Can you work these out from the drawing? Everything is in mm from the part's minimum corner. A direction names the side the tool comes from. Give positions to 0.01 mm unless a question says otherwise; leave off trailing zeros. Write each loop counter-clockwise with the first axis right and the second up, starting at its lowest first coordinate (ties: lowest second). Pieces come first, ordered by that corner, then holes. Notation, with made-up numbers: (34, -33) -> (65, -33) arc R18 ccw to (65, -25) -> close; hole circle Ø10 at (-37, 45). An arc over 180 degrees is marked (long way). Return JSON: item names as keys, results as strings.
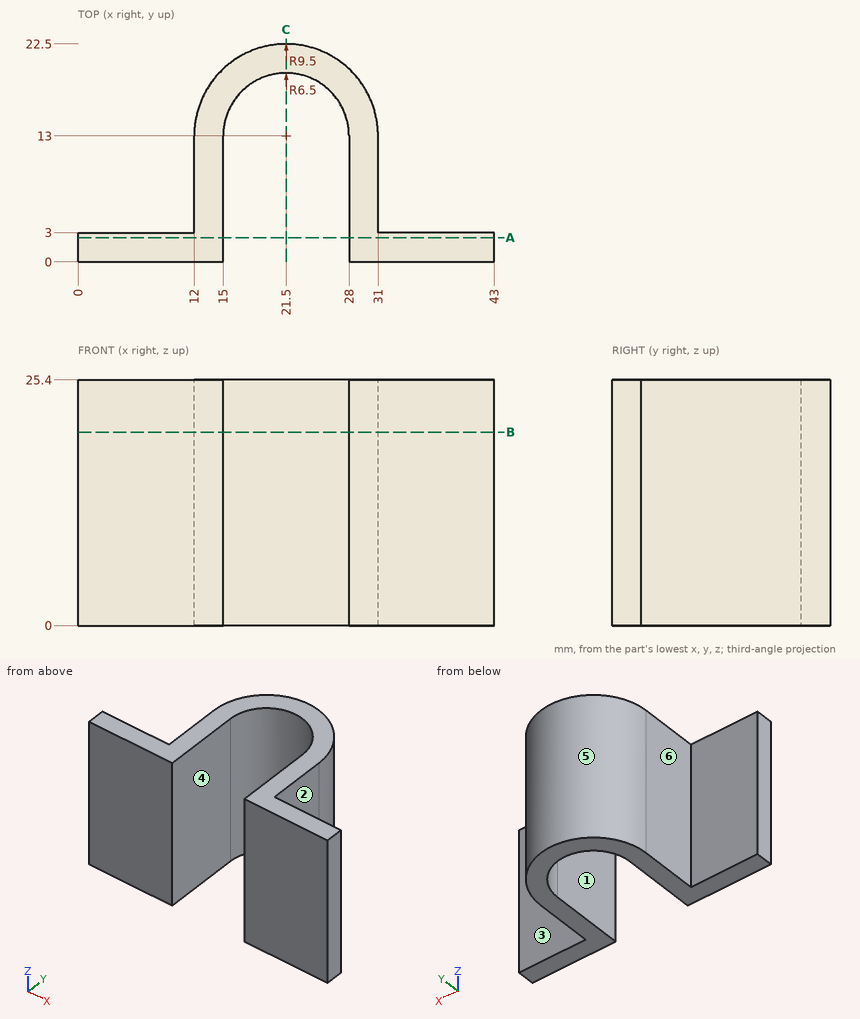
1. Suppose I cut it at C-C, the plane x = 21.5. List the corners of the cut face in (y, z) for me, and give its area (3 significant figures).
Taken from the geometry:
{"outline": "(19.5, 0) -> (22.5, 0) -> (22.5, 25.4) -> (19.5, 25.4) -> close", "area": "76.2 mm²"}
2. If I drill on line 1 (X direction, y = 3.5, z = 8.25); line 2 (Y direction, x = 32, z = 9.5); line 3 (X direction, y = 1, z = 5), over which ranges is the centre line in solid material (lowest first)? Write a range as [from, to].
Taken from the geometry:
{"line 1": "x = [12, 15], [28, 31]", "line 2": "y = [0, 3]", "line 3": "x = [0, 15], [28, 43]"}
3. Suppose I cut it at A-A, the plane y = 2.5. List the corners of the cut face in (x, z) for me, and give its area (3 significant figures).
Taken from the geometry:
{"outline": "(0, 0) -> (15, 0) -> (15, 25.4) -> (0, 25.4) -> close; (28, 0) -> (43, 0) -> (43, 25.4) -> (28, 25.4) -> close", "area": "762 mm²"}
4. Suppose I cut it at B-B, the plane z = 20. List the corners of the cut face in (x, y) for me, and give its area (3 significant figures).
Taken from the geometry:
{"outline": "(0, 0) -> (15, 0) -> (15, 13) arc R6.5 cw to (28, 13) -> (28, 0) -> (43, 0) -> (43, 3) -> (31, 3) -> (31, 13) arc R9.5 ccw to (12, 13) -> (12, 3) -> (0, 3) -> close", "area": "225 mm²"}
5. For pin 1 Ø3 at (y, z) = (8.5, 11) entering from -X; pin 2 Ø11 at (y, z) = (10, 7.5) entering from +X; pin 3 Ø3.5 at (x, z) = (36.5, 6.5) entering from +Y; pin 4 Ø5 at (x, z) = (26.5, 21.5) entering from -Y, each with a flat end and sliding along its axis, tell me the tip position at first contact or that it passes through.
Taken from the geometry:
{"pin 1": "stops at x = 12", "pin 2": "stops at x = 31", "pin 3": "stops at y = 3", "pin 4": "stops at y = 0"}
6. If we mould it in two halves opening along X, with no side actions, what happens to the marked faces 1, 2, 3 and 4? For each: released by +X, released by -X, zero draft, split by the parting line, or undercut.
Taken from the geometry:
{"face 1": "undercut", "face 2": "released by +X", "face 3": "zero draft", "face 4": "undercut"}
7. Which directions (+Z, -Z, +X, -X, +Y, -Y) give clear straight access to the entire face, cutting with the end or side of a thin tool? Please do the marked faces 5 and 6.
Taken from the geometry:
{"face 5": "+Z, -Z, +Y", "face 6": "+Z, -Z, -X, +Y"}
